from build123d import *

# Parameters (mm, degrees)
SKETCH_1_W          = 140
SKETCH_1_H          = 110
EXTRUDE_1_DEPTH     = 3
SKETCH_2_R          = 1.65
CUT_EXTRUDE_1_DEPTH = 90.073003767
SKETCH_3_R          = 1.15
CUT_EXTRUDE_2_DEPTH = 90.073003767
CUT_EXTRUDE_3_DEPTH = 10
CUT_EXTRUDE_4_DEPTH = 10
CUT_EXTRUDE_5_DEPTH = 10
SKETCH_8_R          = 1.6
CUT_EXTRUDE_6_DEPTH = 10


with BuildPart() as part:
    # 草图1 → 凸台-拉伸1 (new body)
    with BuildSketch(Plane.XY):
        Rectangle(SKETCH_1_W, SKETCH_1_H)
    extrude(amount=EXTRUDE_1_DEPTH)

    # 草图2 → 切除-拉伸1 (cut, through all)
    with BuildSketch(Plane(origin=(0, 0, 0), x_dir=(-1, 0, 0), z_dir=(0, 0, -1))):
        with Locations((64, 29)):
            Circle(SKETCH_2_R)
        with Locations((64, -29)):
            Circle(SKETCH_2_R)
        with Locations((49, 29)):
            Circle(SKETCH_2_R)
        with Locations((49, -29)):
            Circle(SKETCH_2_R)
    extrude(amount=-CUT_EXTRUDE_1_DEPTH, mode=Mode.SUBTRACT)

    # 草图3 → 切除-拉伸2 (cut, through all)
    with BuildSketch(Plane(origin=(0, 0, 0), x_dir=(-1, 0, 0), z_dir=(0, 0, -1))):
        with Locations((-40, 7)):
            Circle(SKETCH_3_R)
        with Locations((-40, -7)):
            Circle(SKETCH_3_R)
        with Locations((40, 7)):
            Circle(SKETCH_3_R)
        with Locations((40, -7)):
            Circle(SKETCH_3_R)
    extrude(amount=-CUT_EXTRUDE_2_DEPTH, mode=Mode.SUBTRACT)

    # 草图4 → 切除-拉伸3 (cut)
    with BuildSketch(Plane.XY.offset(3)):
        with BuildLine():
            Line((-25, 42.5), (25, 42.5))
            ThreePointArc((25, 42.5), (27.5, 40), (25, 37.5))
            Line((25, 37.5), (-25, 37.5))
            ThreePointArc((-25, 37.5), (-27.5, 40), (-25, 42.5))
        make_face()
        with BuildLine():
            Line((-25, 26.5), (25, 26.5))
            ThreePointArc((25, 26.5), (27.5, 24), (25, 21.5))
            Line((25, 21.5), (-25, 21.5))
            ThreePointArc((-25, 21.5), (-27.5, 24), (-25, 26.5))
        make_face()
        with BuildLine():
            Line((-25, 10.5), (25, 10.5))
            ThreePointArc((25, 10.5), (27.5, 8), (25, 5.5))
            Line((25, 5.5), (-25, 5.5))
            ThreePointArc((-25, 5.5), (-27.5, 8), (-25, 10.5))
        make_face()
        with BuildLine():
            Line((-25, -5.5), (25, -5.5))
            ThreePointArc((25, -5.5), (27.5, -8), (25, -10.5))
            Line((25, -10.5), (-25, -10.5))
            ThreePointArc((-25, -10.5), (-27.5, -8), (-25, -5.5))
        make_face()
        with BuildLine():
            Line((-25, -21.5), (25, -21.5))
            ThreePointArc((25, -21.5), (27.5, -24), (25, -26.5))
            Line((25, -26.5), (-25, -26.5))
            ThreePointArc((-25, -26.5), (-27.5, -24), (-25, -21.5))
        make_face()
        with BuildLine():
            Line((-25, -37.5), (25, -37.5))
            ThreePointArc((25, -37.5), (27.5, -40), (25, -42.5))
            Line((25, -42.5), (-25, -42.5))
            ThreePointArc((-25, -42.5), (-27.5, -40), (-25, -37.5))
        make_face()
    extrude(amount=-CUT_EXTRUDE_3_DEPTH, mode=Mode.SUBTRACT)

    # 草图5 → 切除-拉伸4 (cut)
    with BuildSketch(Plane.XY.offset(3)):
        with BuildLine():
            Line((-35, 42.5), (35, 42.5))
            ThreePointArc((35, 42.5), (37.5, 40), (35, 37.5))
            Line((35, 37.5), (-35, 37.5))
            ThreePointArc((-35, 37.5), (-37.5, 40), (-35, 42.5))
        make_face()
    cut_extrude_4 = extrude(amount=-CUT_EXTRUDE_4_DEPTH, mode=Mode.SUBTRACT)

    # 镜向1: 切除-拉伸4 across plane
    add(cut_extrude_4.mirror(Plane.ZX), mode=Mode.SUBTRACT)

    # 草图7 → 切除-拉伸5 (cut)
    with BuildSketch(Plane.XY.offset(3)):
        with BuildLine():
            Line((-63, -12.5), (-63, 12.5))
            ThreePointArc((-63, 12.5), (-57, 18.5), (-51, 12.5))
            Line((-51, 12.5), (-51, -12.5))
            ThreePointArc((-51, -12.5), (-57, -18.5), (-63, -12.5))
        make_face()
    extrude(amount=-CUT_EXTRUDE_5_DEPTH, mode=Mode.SUBTRACT)

    # 草图8 → 切除-拉伸6 (cut)
    with BuildSketch(Plane.XY.offset(3)):
        with Locations((55, -48)):
            Circle(SKETCH_8_R)
        with Locations((-55, -48)):
            Circle(SKETCH_8_R)
        with Locations((-55, 48)):
            Circle(SKETCH_8_R)
        with Locations((55, 48)):
            Circle(SKETCH_8_R)
    extrude(amount=-CUT_EXTRUDE_6_DEPTH, mode=Mode.SUBTRACT)


solid = part.part
Read the model definition and answer for the solid it produces. Units are mm, in the model's axes. A direction names the side the tool comes from. Coordinates: 2 decimals unless noted, no trailing zeros. Loops run counter-clockwise (first coordinate to the right, second up) from the corner with the lowest first, then second, coordinate; pieces in that order, holes last.
Q1. The part is cut by section D-D on y = -48. Write down the section's boundary in (x, z).
Q2. Each of these flat-tipped pins is pushed along its axis until it touches: pin 1 Ø1.9 at (x, y) = (-55, 48) entering from -Z; pin 2 Ø2.5 at (x, y) = (-40, 7) entering from +Z. Where does it stop, or does it pass through?
Q3. The part is cut by section C-C on x = -49. Write down the section's boundary in (y, z), and give its area (3 significant figures).
Q4. Consider probe 1 along Y at (x, z) = (-49, 1.4); probe 2 along Y at (x, z) = (32.5, 1.35); probe 3 along X at (y, z) = (-8.5, 1). Determine where each line is inside the solid, lowest interval first.
Q5. Which of the six approach directions +Z, -Z, +X, -X, +Y, -Y give full straight-line access (tool end or side, diameter ignored) to faces 1 (the face through (-37.5, 39.9, 1.5)), 2 (the face through (-1, 55, 1))?
Q6. The mould has two halves that part along X. Classify faces 3 (the face through (37.5, -40.1, 1.5)), 4 (the face through (-1, 1, 3)): +X half, -X half, draft (parallel to the pull), parting line (faces both ways), or undercut.
Q7. The part is cut by section A-A on x = -1. Write down the section's boundary in (y, z).
Q8. The part is cut by section B-B on y = 40. Write down the section's boundary in (x, z).
Results below:
1. outline: (-70, 0) - (-56.6, 0) - (-56.6, 3) - (-70, 3) - close; (-53.4, 0) - (53.4, 0) - (53.4, 3) - (-53.4, 3) - close; (56.6, 0) - (70, 0) - (70, 3) - (56.6, 3) - close
2. pin 1: passes through
2. pin 2: stops at z = 3
3. outline: (-55, 0) - (-30.65, 0) - (-30.65, 3) - (-55, 3) - close; (-27.35, 0) - (27.35, 0) - (27.35, 3) - (-27.35, 3) - close; (30.65, 0) - (55, 0) - (55, 3) - (30.65, 3) - close
3. area: 310 mm2
4. probe 1: y = -55 to -30.65, -27.35 to 27.35, 30.65 to 55
4. probe 2: y = -55 to -42.5, -37.5 to 37.5, 42.5 to 55
4. probe 3: x = -70 to -63, -51 to -27.45, 27.45 to 70
5. face 1: +Z, -Z
5. face 2: +Z, -Z, +X, -X, +Y
6. face 3: undercut
6. face 4: draft
7. outline: (-55, 0) - (-42.5, 0) - (-42.5, 3) - (-55, 3) - close; (-37.5, 0) - (-26.5, 0) - (-26.5, 3) - (-37.5, 3) - close; (-21.5, 0) - (-10.5, 0) - (-10.5, 3) - (-21.5, 3) - close; (-5.5, 0) - (5.5, 0) - (5.5, 3) - (-5.5, 3) - close; (10.5, 0) - (21.5, 0) - (21.5, 3) - (10.5, 3) - close; (26.5, 0) - (37.5, 0) - (37.5, 3) - (26.5, 3) - close; (42.5, 0) - (55, 0) - (55, 3) - (42.5, 3) - close
8. outline: (-70, 0) - (-37.5, 0) - (-37.5, 3) - (-70, 3) - close; (37.5, 0) - (70, 0) - (70, 3) - (37.5, 3) - close
